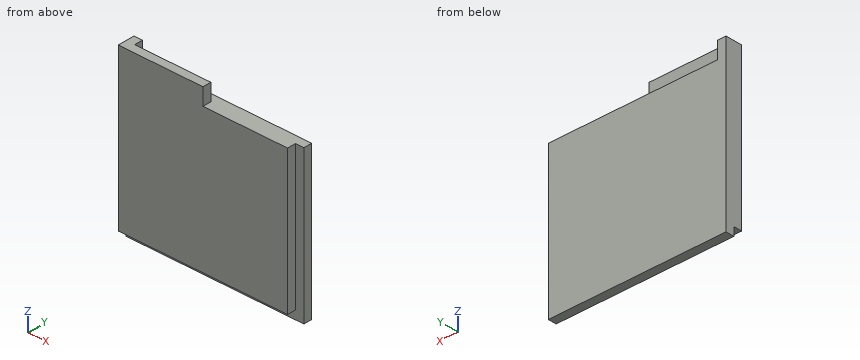
from build123d import *

# Parameters (mm, degrees)
F0_W      = 105
F0_H      = 95
F1_DEPTH  = 5
F2_W      = 50
F2_H      = 5
F3_DEPTH  = 5
F5_DEPTH  = 5
F6_W      = 5
F6_H      = 5
F7_DEPTH  = 45
F8_W      = 10
F8_H      = 5
F9_DEPTH  = 5
F9_FACE_W = 5
F9_FACE_H = 5
F10_DEPTH = 90


with BuildPart() as f1:
    # F0 (on Front) → F1 (new body)
    with BuildSketch(Plane.XZ):
        Rectangle(F0_W, F0_H)
    extrude(amount=F1_DEPTH)

    # F2 (on face) → F3 (join)
    with BuildSketch(Plane.XY.offset(47.5)):
        with Locations((-27.5, -2.5)):
            Rectangle(F2_W, F2_H)
    extrude(amount=F3_DEPTH)

    # F4 (on face) → F5 (join)
    with BuildSketch(Plane.XZ.offset(5)):
        Polygon((-2.5, 42.5), (-2.5, 47.5), (-2.5, 52.5), (-52.5, 52.5), (-52.5, -42.5), (47.5, -42.5), (47.5, 42.5), align=None)
    extrude(amount=F5_DEPTH)

    # F6 (on face) → F7 (cut)
    with BuildSketch(Plane.YZ.offset(-2.5)):
        with Locations((-2.5, 50)):
            Rectangle(F6_W, F6_H)
    extrude(amount=-F7_DEPTH, mode=Mode.SUBTRACT)

    # F8 (on face) → F9 (cut)
    with BuildSketch(Plane.XY.offset(47.5)):
        with Locations((-42.5, -2.5)):
            Rectangle(F8_W, F8_H)
    extrude(amount=-F9_DEPTH, mode=Mode.SUBTRACT)

    # F9_face (on face) → F10 (cut)
    with BuildSketch(Plane(origin=(-37.5, -2.5, 45), x_dir=(0, -1, 0), z_dir=(-1, 0, 0))):
        Rectangle(F9_FACE_W, F9_FACE_H)
    extrude(amount=-F10_DEPTH, mode=Mode.SUBTRACT)


solid = f1.part
Model file for the job. Use its own axes, mm. Coordinates: 2 decimals unless noted, no trailing zeros. Write each loop counter-clockwise with the first axis right and the second up, starting at its lowest first coordinate (ties: lowest second). Pieces come first, ordered by that corner, then holes. Notation, with made-up numbers: (-20, 42) -> (23, 42) arc R24 ccw to (23, 79) -> close; hole circle Ø7 at (50, 42.25). An arc over 180 degrees is marked (long way). One line per item, written item: value. Start each with the question number.
1) Slice it at B-B on z = 14. Write the cut outline in (x, y), then the cut area to 4 significant figures.
2) Slice it at A-A on y = -8.25. Write the cut outline in (x, z), then the cut area to 3 significant figures.
3) Probe probe 1 along Z at (x, y) = (-0.5, -7.25); probe 2 along Z at (x, y) = (-38, -9.5); probe 3 along X at (y, z) = (-7.75, -15.5). List the from-to ranges inside material, lowest first.
4) Flat gauge pins, fed straight in: pin 1 Ø4 at (y, z) = (-8.5, 49.5) entering from +X; pin 2 Ø1.5 at (y, z) = (-6.5, 9) entering from +X; pin 3 Ø3 at (x, y) = (26.5, -5) entering from +Z. Where does each tip first touch, or does it go through?
5) Slice it at C-C on x = -27. Write the cut outline in (y, z), then the cut area to 3 significant figures.
Answers follow:
1. outline: (-52.5, -10) -> (47.5, -10) -> (47.5, -5) -> (52.5, -5) -> (52.5, 0) -> (-52.5, 0) -> close
1. area: 1,025 mm2
2. outline: (-52.5, -42.5) -> (47.5, -42.5) -> (47.5, 42.5) -> (-2.5, 42.5) -> (-2.5, 52.5) -> (-52.5, 52.5) -> close
2. area: 9,000 mm2
3. probe 1: -42.5 to 42.5
3. probe 2: -42.5 to 52.5
3. probe 3: -52.5 to 47.5
4. pin 1: x = -2.5
4. pin 2: x = 47.5
4. pin 3: z = 42.5
5. outline: (-10, -42.5) -> (-5, -42.5) -> (-5, -47.5) -> (0, -47.5) -> (0, 42.5) -> (-5, 42.5) -> (-5, 52.5) -> (-10, 52.5) -> close
5. area: 925 mm2
